from build123d import *

# Parameters (mm, degrees)
EXTRUDE_1_DEPTH     = 4
CUT_EXTRUDE_1_REACH = 66.946
SKETCH_2_R          = 2
SKETCH_2_R_2        = 2.1
FILLET_1_R          = 2


with BuildPart() as part:
    # 草图1 → 凸台-拉伸1 (new body)
    with BuildSketch(Plane.XY):
        with BuildLine():
            Line((22.535898385, 60), (-20, 60))
            Line((-20, 60), (-20, 30))
            Line((-20, 30), (-20, -30))
            Line((-20, -30), (20, -30))
            Line((20, -30), (20, 30))
            Line((20, 30), (7.749348907, 37.54075723))
            Line((7.749348907, 37.54075723), (7.749348907, 47.153580602))
            Line((7.749348907, 47.153580602), (23.535898385, 56.267949192))
            ThreePointArc((23.535898385, 56.267949192), (24.467750037, 58.51763809), (22.535898385, 60))
        make_face()
    extrude(amount=EXTRUDE_1_DEPTH)

    # 草图2 → 切除-拉伸1 (cut, up to next)
    with BuildSketch(Plane.XY.offset(4), mode=Mode.PRIVATE) as cut_extrude_1_sk1:
        with Locations((-10, -24.5)):
            Circle(SKETCH_2_R)
    cut_extrude_1_tool1 = extrude(cut_extrude_1_sk1.sketch, amount=-CUT_EXTRUDE_1_REACH, mode=Mode.PRIVATE) & part.part
    # 草图2 → 切除-拉伸1 (cut, up to next)
    with BuildSketch(Plane.XY.offset(4), mode=Mode.PRIVATE) as cut_extrude_1_sk2:
        with Locations((-10, -10.5)):
            Circle(SKETCH_2_R_2)
    cut_extrude_1_tool2 = extrude(cut_extrude_1_sk2.sketch, amount=-CUT_EXTRUDE_1_REACH, mode=Mode.PRIVATE) & part.part
    # 草图2 → 切除-拉伸1 (cut, up to next)
    with BuildSketch(Plane.XY.offset(4), mode=Mode.PRIVATE) as cut_extrude_1_sk3:
        with Locations((10, -10.5)):
            Circle(SKETCH_2_R_2)
    cut_extrude_1_tool3 = extrude(cut_extrude_1_sk3.sketch, amount=-CUT_EXTRUDE_1_REACH, mode=Mode.PRIVATE) & part.part
    # 草图2 → 切除-拉伸1 (cut, up to next)
    with BuildSketch(Plane.XY.offset(4), mode=Mode.PRIVATE) as cut_extrude_1_sk4:
        with Locations((10, -24.5)):
            Circle(SKETCH_2_R)
    cut_extrude_1_tool4 = extrude(cut_extrude_1_sk4.sketch, amount=-CUT_EXTRUDE_1_REACH, mode=Mode.PRIVATE) & part.part
    add(cut_extrude_1_tool1.solids().sort_by_distance((-10, -24.5, 4))[0], mode=Mode.SUBTRACT)
    add(cut_extrude_1_tool2.solids().sort_by_distance((-10, -10.5, 4))[0], mode=Mode.SUBTRACT)
    add(cut_extrude_1_tool3.solids().sort_by_distance((10, -10.5, 4))[0], mode=Mode.SUBTRACT)
    add(cut_extrude_1_tool4.solids().sort_by_distance((10, -24.5, 4))[0], mode=Mode.SUBTRACT)

    # 圆角1
    fillet_1_edges = [part.edges().sort_by_distance(p)[0] for p in [
        (20, 30, 2),
        (20, -30, 2),
        (-20, -30, 2),
        (-20, 60, 2),
    ]]
    fillet(fillet_1_edges, radius=FILLET_1_R)


solid = part.part
Read the model definition and answer for the solid it produces. Units are mm, in the model's axes. A direction names the side the tool comes from. Coordinates: 2 decimals unless noted, no trailing zeros. Write each loop counter-clockwise with the first axis right and the second up, starting at its lowest first coordinate (ties: lowest second). Pieces come first, ordered by that corner, then holes. Notation, with made-up numbers: M 64,49.5 L 72,49.5 A19 cw 72,72.5 Z; hole C 6.25,40.5 d3. An arc over 180 degrees is marked long. Use a Markdown table: item, result.
Q1. Which of the six approach directions +Z, -Z, +X, -X, +Y, -Y give full straight-line access (tool end or side, diameter ignored) to faces 1 (the face through (-19.43, -29.4, 2.03)), 2 (the face through (7.749, 42, 2)), 3 (the face through (20, 0, 2))?
Answer block:
| item | result |
|---|---|
| face 1 | +Z, -Z, -X, -Y |
| face 2 | +Z, -Z, +X |
| face 3 | +Z, -Z, +X, -Y |
Q2. The part is cut by section C-C, the plane x = -10. Write down the section's boundary in (y, z), then the cut area to 3 significant figures.
Answer block:
| item | result |
|---|---|
| outline | M -30,0 L -26.5,0 L -26.5,4 L -30,4 Z; M -22.5,0 L -12.6,0 L -12.6,4 L -22.5,4 Z; M -8.4,0 L 60,0 L 60,4 L -8.4,4 Z |
| area | 327 mm2 |
Q3. The part is cut by section A-A, the plane y = -10.5. Write down the section's boundary in (x, z), then the cut area to 3 significant figures.
Answer block:
| item | result |
|---|---|
| outline | M -20,0 L -12.1,0 L -12.1,4 L -20,4 Z; M -7.9,0 L 7.9,0 L 7.9,4 L -7.9,4 Z; M 12.1,0 L 20,0 L 20,4 L 12.1,4 Z |
| area | 126 mm2 |
Q4. Straight lines are drawn through the part: L1, parallel to Y at x = -10, z = 1.1; L2, parallel to Y at x = 10, z = 1.25; L3, parallel to X at y = -8, z = 0.9. For each, find the intervals that lie inside material, in ascending order. Write a range as [from, to].
Answer block:
| item | result |
|---|---|
| L1 | y = [-30, -26.5], [-22.5, -12.6], [-8.4, 60] |
| L2 | y = [-30, -26.5], [-22.5, -12.6], [-8.4, 36.16], [48.45, 60] |
| L3 | x = [-20, 20] |
Q5. Determine the mould class of faces 4 (the face through (7.9, -10.41, 2.03)), 5 (the face through (24.477, 58.482, 1.972)), 6 (the face through (8.4, -25.7, 2)), 7 (the face through (-19.4, 59.43, 2.03)) for opening direction X: released by +X, released by -X, zero draft, split by the parting line, or undercut.
Answer block:
| item | result |
|---|---|
| face 4 | undercut |
| face 5 | released by +X |
| face 6 | undercut |
| face 7 | released by -X |
Q6. The part is cut by section D-D, the plane x = 10. Write down the section's boundary in (y, z).
Answer block:
| item | result |
|---|---|
| outline | M -30,0 L -26.5,0 L -26.5,4 L -30,4 Z; M -22.5,0 L -12.6,0 L -12.6,4 L -22.5,4 Z; M -8.4,0 L 36.16,0 L 36.16,4 L -8.4,4 Z; M 48.45,0 L 60,0 L 60,4 L 48.45,4 Z |
Q7. Each of these flat-tipped pins is pushed along its axis until it touches: pin 1 Ø1.5 at (y, z) = (0, 1.5) entering from +X; pin 2 Ø2.5 at (x, y) = (10, -24.5) entering from -Z. Where does it stop, or does it pass through?
Answer block:
| item | result |
|---|---|
| pin 1 | stops at x = 20 |
| pin 2 | passes through |
Q8. The part is cut by section B-B, the plane z = 3.2. Write down the section's boundary in (x, y), then the cut area to 3 significant figures.
Answer block:
| item | result |
|---|---|
| outline | M -20,-28 A2 ccw -18,-30 L 18,-30 A2 ccw 20,-28 L 20,28.88 A2 ccw 19.05,30.59 L 7.75,37.54 L 7.75,47.15 L 23.54,56.27 A2 ccw 22.54,60 L -18,60 A2 ccw -20,58 Z; hole C -10,-10.5 d4.2; hole C -10,-24.5 d4; hole C 10,-10.5 d4.2; hole C 10,-24.5 d4 |
| area | 3,360 mm2 |
